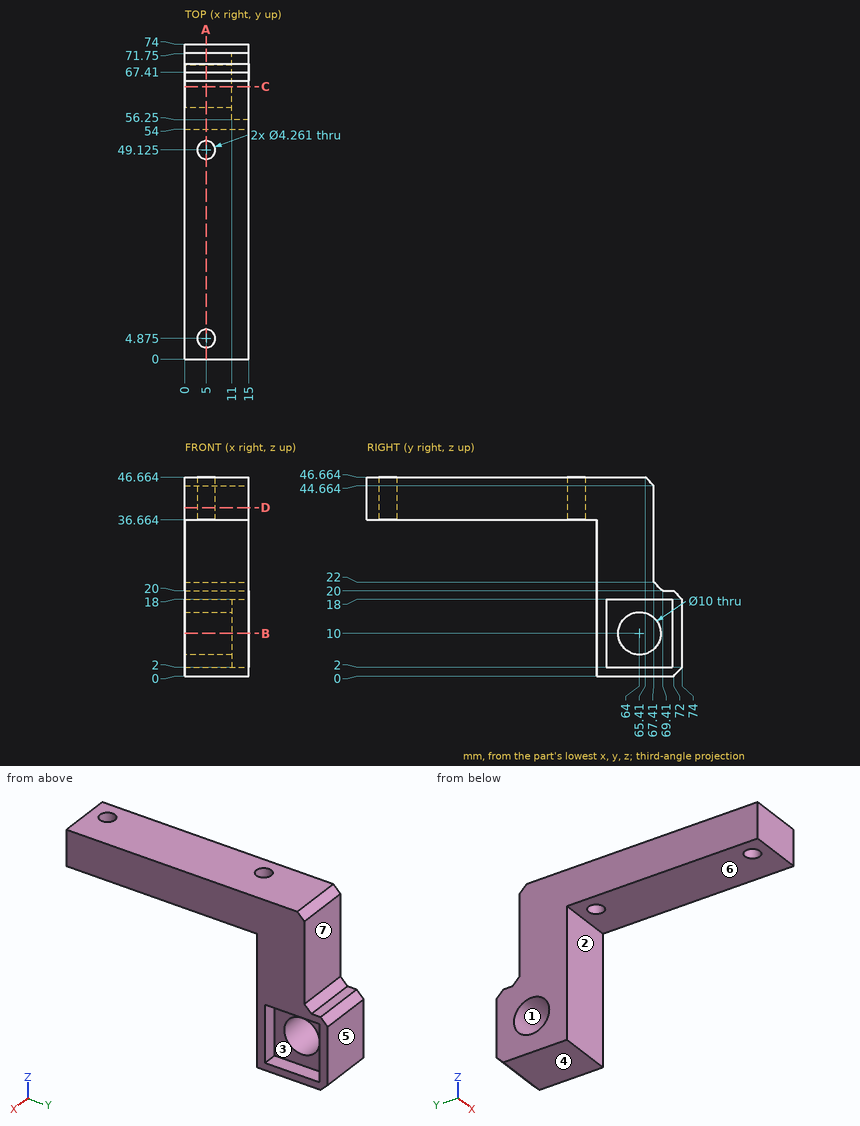
The drawing under review shows one solid part. Ordinate dimensions are in mm from its lowest x, y, z. A direction names the side the tool comes from. Coordinates: 2 decimals unless noted, no trailing zeros. Write each loop counter-clockwise with the first axis right and the second up, starting at its lowest first coordinate (ties: lowest second). Pieces come first, ordered by that corner, then holes. Notation, with made-up numbers: (75, 65.25) - (90, 65.25) arc R15 cw to (90, 82.25) - close; hole circle Ø11 at (32, 33). An arc over 180 degrees is marked (long way). Put each result on its own line as item: value.
1. Machinability: for the marked faces 5, 6 and 7, which of the approach directions +Z, -Z, +X, -X, +Y, -Y give a long, thin tool a straight path to every point of the face, cutting with its end or side? Answer none if there is none.
Values found:
face 5: +Z, -Z, +X, -X, +Y
face 6: -Z, +X, -X, -Y
face 7: +Z, +X, -X, +Y
2. Add section D-D, the plane z = 39.5. Give the boundary of the cut face in (x, y) (1 decimal).
Values found:
outline: (0, 0) - (15, 0) - (15, 67.4) - (0, 67.4) - close; hole circle Ø4.3 at (5, 4.9); hole circle Ø4.3 at (5, 49.1)
3. Mouldability with a two-part tool opening along Y and no side actions: class the marked faces 1, 2, 3 and 4 as released by +Y, released by -Y, zero draft, split by the parting line, or undercut.
Values found:
face 1: undercut
face 2: released by -Y
face 3: undercut
face 4: zero draft
4. Wall thickness on probe 1 along Y at (x, z) = (5, 43.5) (1 decimal); probe 2 along Y at (x, z) = (2.5, 10); probe 3 along Z at (x, y) = (14, 58.5) (1 decimal): over which ranges is each line inside the solid? List them lowest first.
Values found:
probe 1: 0 to 2.7, 7 to 47, 51.3 to 67.4
probe 2: 54 to 59, 69 to 74
probe 3: 0 to 2, 18 to 46.7
5. For pin 1 (4.5 mm diameter, centred on x = 13.5, z = 11, fed in from -Y); pin 2 (10 mm diameter, centred on y = 55.5, z = 9.5, fed in from -X); pin 3 (1.3 mm diameter, centred on x = 6.5, y = 70.5, fed in from +Z); pin 4 (1.5 mm diameter, centred on x = 5.5, z = 26, fed in from +Y), all flat-tipped, find the tip position at first contact; note any pin that passes through.
Values found:
pin 1: y = 54
pin 2: x = 0
pin 3: z = 20
pin 4: y = 67.41
6. Add section B-B, the plane z = 10. Give the boundary of the cut face in (x, y), then the cut area to 3 significant figures.
Values found:
outline: (0, 54) - (15, 54) - (15, 56.25) - (11, 56.25) - (11, 59) - (0, 59) - close; (0, 69) - (11, 69) - (11, 71.75) - (15, 71.75) - (15, 74) - (0, 74) - close
area: 128 mm²
7. Add section C-C, the plane y = 64. Give the boundary of the cut face in (x, z) (1 decimal), then the cut area to 3 significant figures.
Values found:
outline: (0, 0) - (15, 0) - (15, 2) - (11, 2) - (11, 5) - (0, 5) - close; (0, 15) - (11, 15) - (11, 18) - (15, 18) - (15, 46.7) - (0, 46.7) - close
area: 526 mm²
8. Add section A-A, the plane x = 5. Give the boundary of the cut face in (y, z) (1 decimal), then the cut area to 3 significant figures.
Values found:
outline: (0, 36.7) - (2.7, 36.7) - (2.7, 46.7) - (0, 46.7) - close; (7, 36.7) - (47, 36.7) - (47, 46.7) - (7, 46.7) - close; (51.3, 36.7) - (54, 36.7) - (54, 0) - (72, 0) - (74, 2) - (74, 18) - (72, 20) - (69.4, 20) - (67.4, 22) - (67.4, 44.7) - (65.4, 46.7) - (51.3, 46.7) - close; hole circle Ø10 at (64, 10)
area: 1,130 mm²
